Source: three-view drawing plus pictorial views. Frame: mm from the lowest corner of the part. A direction names the side the tool comes from. Coordinates: 2 decimals unless noted, no trailing zeros. Loops run counter-clockwise (first coordinate to the right, second up) from the corner with the lowest first, then second, coordinate; pieces in that order, holes last. Notation, with made-up numbers: (4, 17) - (22, 17) arc R29 ccw to (22, 39) - close; hole circle Ø5 at (63, -1). An arc over 180 degrees is marked (long way). Use CSV: the item, a comma, the result in double quotes. Start each with the question number.
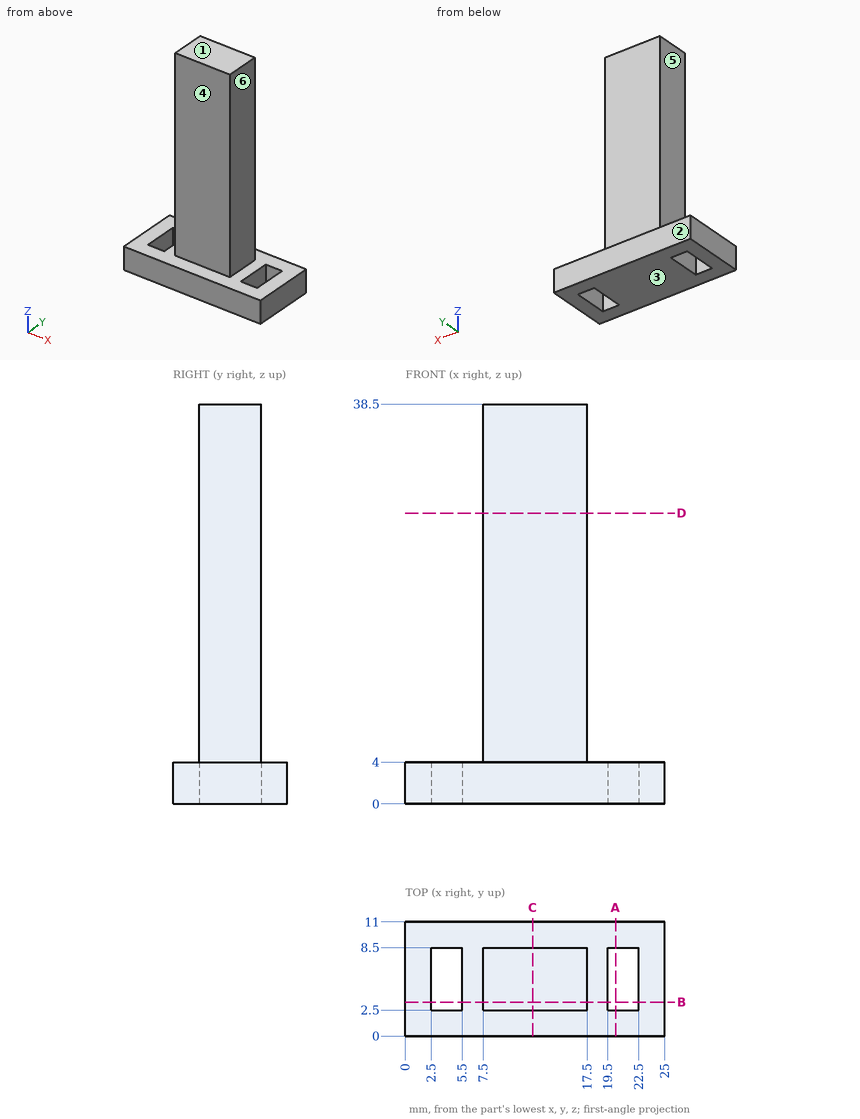
(1) Section D-D on z = 28. Output: boundary loops of the cut face in (x, y).
(2) Draft query along Z for the marked faces 1, 2 and 3. Return one class per face: released by +Z, released by -Z, zero draft, split by the parting line, or undercut.
(3) Ray query, line 1 (X direction, y = 7.5, z = 27); line 2 (Z direction, x = 23.75, y = 6); line 3 (Y direction, x = 9.25, z = 18). Return the intervals inside material, ascending. Write a range as [from, to].
(4) Section A-A on x = 20.25. Output: boundary loops of the cut face in (y, z), plus the area to 3 significant figures.
(5) Section B-B on y = 3.25. Output: boundary loops of the cut face in (x, z), plus the area to 3 significant figures.
(6) Reachability of the marked faces 4, 5 and 6 from +Z, -Z, +X, -X, +Y, -Y: full face, straight path, thin tool, end or side. Return the list, or none.
(7) Section C-C on x = 12.25. Output: boundary loops of the cut face in (y, z), plus the area to 3 significant figures.
(8) Pin query (flat end, axial travel): pin 1 Ø5 at (y, z) = (7, 19) entering from -X; pin 2 Ø11 at (x, z) = (13, 15.5) entering from +Y; pin 3 Ø2 at (y, z) = (5, 1) entering from -X; pin 4 Ø1.8 at (y, z) = (5, 21) entering from +X. Return the tip coordinate at first contact, or that it passes through.
Solution:
1,outline,"(7.5, 2.5) - (17.5, 2.5) - (17.5, 8.5) - (7.5, 8.5) - close"
2,face 1,"released by +Z"
2,face 2,"zero draft"
2,face 3,"released by -Z"
3,line 1,"x = [7.5, 17.5]"
3,line 2,"z = [0, 4]"
3,line 3,"y = [2.5, 8.5]"
4,outline,"(0, 0) - (2.5, 0) - (2.5, 4) - (0, 4) - close; (8.5, 0) - (11, 0) - (11, 4) - (8.5, 4) - close"
4,area,"20.0 mm²"
5,outline,"(0, 0) - (2.5, 0) - (2.5, 4) - (0, 4) - close; (5.5, 0) - (19.5, 0) - (19.5, 4) - (17.5, 4) - (17.5, 38.5) - (7.5, 38.5) - (7.5, 4) - (5.5, 4) - close; (22.5, 0) - (25, 0) - (25, 4) - (22.5, 4) - close"
5,area,"421 mm²"
6,face 4,"+Z, +X, -X, -Y"
6,face 5,"+Z, -X, +Y, -Y"
6,face 6,"+Z, +X, +Y, -Y"
7,outline,"(0, 0) - (11, 0) - (11, 4) - (8.5, 4) - (8.5, 38.5) - (2.5, 38.5) - (2.5, 4) - (0, 4) - close"
7,area,"251 mm²"
8,pin 1,"stops at x = 7.5"
8,pin 2,"stops at y = 8.5"
8,pin 3,"stops at x = 0"
8,pin 4,"stops at x = 17.5"
